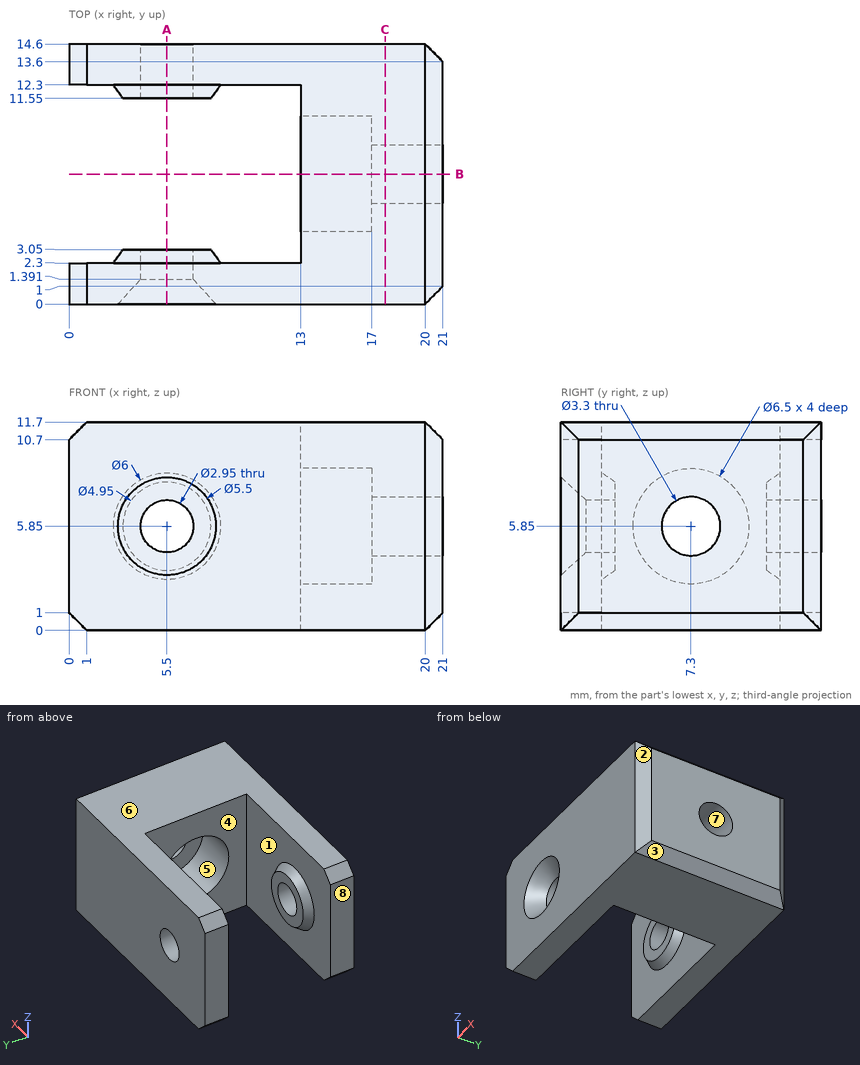
Could you check a few things on this drawing? It's one solid part, dimensions in mm from its lowest x, y, z. A direction names the side the tool comes from. Round coordinates to 2 decimals unless told otherwise and drop trailing zeros. Order: outer loops, then holes, each group sorted by start corner. A loop starts at its lowest first (then second) coordinate and runs counter-clockwise, first axis right, second up. Notation, with made-up numbers: (52, -10.5) -> (72, -10.5) arc R19 cw to (72, 2.5) -> close; hole circle Ø8 at (24.25, 34.5). An arc over 180 degrees is marked (long way). One line per question, with ' | ' between items.
Q1. If we section it at C-C on x = 17.75: Write out the boundary of the cut face in (y, z), plus the area to 3 significant figures.
Computed values:
outline: (0, 0) -> (14.6, 0) -> (14.6, 11.7) -> (0, 11.7) -> close; hole circle Ø3.3 at (7.3, 5.85) | area: 162 mm²
Q2. If I drill on line 1 (Z direction, x = 5.5, y = 12.85) (1 decimal); line 2 (Y direction, x = 11.5, z = 1); line 3 (X direction, y = 3.75, z = 8), over which ranges is the centre line in solid material (lowest first)? Write a range as from..to.
Computed values:
line 1: 0..4.4, 7.3..11.7 | line 2: 0..2.3, 12.3..14.6 | line 3: 13..21
Q3. If we section it at B-B on y = 7.3: Write out the boundary of the cut face in (x, z).
Computed values:
outline: (13, 0) -> (20, 0) -> (21, 1) -> (21, 4.2) -> (17, 4.2) -> (17, 2.6) -> (13, 2.6) -> close; (13, 9.1) -> (17, 9.1) -> (17, 7.5) -> (21, 7.5) -> (21, 10.7) -> (20, 11.7) -> (13, 11.7) -> close
Q4. We'd pull the mould along Z, two halves only. Please class the marked faces 6, 7 and 8: released by +Z, released by -Z, zero draft, split by the parting line, or undercut.
Computed values:
face 6: released by +Z | face 7: undercut | face 8: zero draft
Q5. Which directions (+Z, -Z, +X, -X, +Y, -Y) give clear straight access to the entire face, cutting with the end or side of a thin tool? Please do the marked faces 1, 2, 3, 4 and 5.
Computed values:
face 1: none | face 2: +Z, -Z, +X, -Y | face 3: -Z, +X, +Y, -Y | face 4: +Z, -Z | face 5: -X
Q6. I'm going to push flat-ended pins straight in: pin 1 (4 mm diameter, centred on y = 7.3, z = 5.85, fed in from -X); pin 2 (2.5 mm diameter, centred on x = 5.5, z = 5.85, fed in from +Y); pin 3 (1.5 mm diameter, centred on x = 4.5, z = 6.5, fed in from -Y); pin 4 (5 mm diameter, centred on y = 8, z = 5.5, fed in from -X). Where does each tip first touch, or does it pass through?
Computed values:
pin 1: x = 17 | pin 2: through | pin 3: y = 0.88 | pin 4: x = 13
Q7. If we section it at A-A on x = 5.5: Give the number of separate pieces and of enclosed holes in the cut face.
Computed values:
separate pieces: 4 | enclosed holes: 0
